Design review of the part built by this model. Coordinates are the model's own, in mm. A direction names the side the tool comes from. Coordinates: 2 decimals unless noted, no trailing zeros. Write each loop counter-clockwise with the first axis right and the second up, starting at its lowest first coordinate (ties: lowest second). Pieces come first, ordered by that corner, then holes.
Q1. Take a section at C-C, the plane x = 22. Write out the cut boundary in (y, z), plus the area to 3 significant figures.
Q2. For faces 1 (the flat face through (23, 0.833, 3)), 2 (the flat face through (0, 23, 3)), list the 3-axis set-ups (+Z, -Z, +X, -X, +Y, -Y) from which the entire face can be reached by the end or side of a thin tool; tool diameter is ignored.
Q3. For L1, parallel to X at y = 40.5, z = -53.5, list the stretches that pass through material, from the lowest coordinate up.
Q4. Take a section at B-B, the plane y = 16. Write out the cut boundary in (x, z).
Q5. For pin 1 Ø3 at (y, z) = (18, -88) entering from +X; pin 2 Ø2 at (x, z) = (21.5, 141) entering from +Y, all flat-tipped, find the tip position at first contact; note any pin that passes through.
Q6. Take a section at A-A, the plane z = -136. Write out the cut boundary in (x, y).
from build123d import *

# Parameters (mm, degrees)
BOSS_EXTRUDE1_DEPTH = 210


with BuildPart() as part:
    # Sketch1 → Boss-Extrude1 (new, symmetric)
    with BuildSketch(Plane.XY):
        Polygon((0, 45), (0, 0), (45, 0), (45, 0.833333333), (0.833333333, 0.833333333), (0.833333333, 45), align=None)
    extrude(amount=BOSS_EXTRUDE1_DEPTH, both=True)

    # SurfaceCut5
    split(bisect_by=Plane(origin=(100.416666667, 0, -100.416666667), x_dir=(0.7071067811865487, 0, 0.7071067811865465), z_dir=(-0.7071067811865465, 0, 0.7071067811865487)), keep=Keep.TOP)

    # SurfaceCut6
    split(bisect_by=Plane(origin=(100.416666667, 0, 100.416666667), x_dir=(0.7071067811865487, 0, -0.7071067811865465), z_dir=(0.7071067811865465, 0, 0.7071067811865487)), keep=Keep.BOTTOM)


solid = part.part
Responses:
1. outline: (0, -178.83) - (0.83, -178.83) - (0.83, 178.83) - (0, 178.83) - close
1. area: 298 mm2
2. face 1: +Z, -Z, +X, +Y
2. face 2: +Z, -Z, -X, +Y, -Y
3. L1: x = 0 to 0.83
4. outline: (0, -200.83) - (0.83, -200) - (0.83, 200) - (0, 200.83) - close
5. pin 1: stops at x = 0.83
5. pin 2: stops at y = 0.83
6. outline: (0, 0) - (45, 0) - (45, 0.83) - (0.83, 0.83) - (0.83, 45) - (0, 45) - close
